```python
from build123d import *

# Parameters (mm, degrees)
CHANFREIN1_SIZE           = 0.5
CHANFREIN2_SIZE           = 1
TROU_TARAUD_M8X1_01_D     = 7
TROU_TARAUD_M8X1_01_DEPTH = 23
TROU_TARAUD_M8X1_01_TIP   = 2.103012167


with BuildPart() as part:
    # Esquisse1 → Révolution1 (revolve)
    with BuildSketch(Plane.XY, mode=Mode.PRIVATE) as r_volution1_sk:
        Polygon((-44, 23), (-13, 23), (-13, 20), (13, 20), (13, 18), (56, 18), (56, 17), (60.5, 17), (60.5, 12.5), (76.5, 12.5), (76.5, 0), (-44, 0), align=None)
    revolve(r_volution1_sk.sketch.rotate(Axis((-47.210983023, 0, 0), (1, 0, 0)), 90), axis=Axis((-47.210983023, 0, 0), (1, 0, 0)))

    # Chanfrein1
    chanfrein1_edges = [part.edges().sort_by_distance(p)[0] for p in [
        (56, 0, -18),
        (13, 0, -20),
        (-13, 0, -23),
    ]]
    chamfer(chanfrein1_edges, length=CHANFREIN1_SIZE)

    # Chanfrein2
    chanfrein2_edges = [part.edges().sort_by_distance(p)[0] for p in [
        (76.5, 0, -12.5),
    ]]
    chamfer(chanfrein2_edges, length=CHANFREIN2_SIZE)

    # Trou taraudé M8x1.01
    with Locations(Plane(origin=(76.5, 0, 0), x_dir=(0, 0, -1), z_dir=(1, 0, 0))):
        with Locations((0, 0)):
            Hole(TROU_TARAUD_M8X1_01_D / 2, depth=TROU_TARAUD_M8X1_01_DEPTH)
            with Locations((0, 0, -(TROU_TARAUD_M8X1_01_DEPTH + TROU_TARAUD_M8X1_01_TIP / 2))):  # 118° drill point
                Cone(0, TROU_TARAUD_M8X1_01_D / 2, TROU_TARAUD_M8X1_01_TIP, mode=Mode.SUBTRACT)


solid = part.part
```
Can you work these out from the model? Positions are in its coordinate system, mm. A direction names the side the tool comes from. Coordinates: 2 decimals unless noted, no trailing zeros. Order: outer loops, then holes, each group sorted by start corner. A loop starts at its lowest first (then second) coordinate and runs counter-clockwise, first axis right, second up. Notation, with made-up numbers: (71.5, 20.5) -> (77.5, 20.5) arc R30 cw to (77.5, 42.5) -> close; hole circle Ø10 at (23, 70.25). An arc over 180 degrees is marked (long way). Write each question's results on one line, items separated by ' | '.
Item 1: Which directions (+Z, -Z, +X, -X, +Y, -Y) give clear straight access to the entire face, cutting with the end or side of a thin tool? Please do faces 4 (the face through (58.282, -16.855, -2.213)), 5 (the face through (76.5, -3, -3)).
Results are:
face 4: +X | face 5: +Z, -Z, +X, +Y, -Y
Item 2: I'm going to push flat-ended pins straight in: pin 1 Ø1 at (x, y) = (-4.5, -2.5) entering from +Z; pin 2 Ø8 at (x, z) = (30, 6) entering from -Y; pin 3 Ø12 at (x, y) = (10.5, 1) entering from +Z. Where does each tip first touch, or does it pass through?
Results are:
pin 1: z = 19.9 | pin 2: y = -17.89 | pin 3: z = 20
Item 3: If I drill on line 1 along Y through (x, z) = (58.25, 0); line 2 along Y through (x, z) = (62, 0); line 3 along X through (y, z) = (-7.5, 20.5), over which ranges is the centre line in solid material (lowest first)?
Results are:
line 1: -17 to -3.5, 3.5 to 17 | line 2: -12.5 to -3.5, 3.5 to 12.5 | line 3: -44 to -13
Item 4: If we mould it in two halves opening along Y, with no side actions, what happens to faces 1 (the face through (64.839, -1.341, 3.233)), 2 (the face through (-28.536, -22.804, -2.994)), 3 (the face through (-13, 1.6, -20.1))? For each: +Y half, -Y half, draft (parallel to the pull), parting line (faces both ways), or undercut.
Results are:
face 1: undercut | face 2: parting line | face 3: draft
Item 5: I want a section at A-A, the plane x = 24. Write out the boundary of the cut face in (y, z).
Results are:
outline: circle Ø36 at (0, 0)
Item 6: I want a section at B-B, the plane x = -18.5. Write out the boundary of the cut face in (y, z), then the cut area to 3 significant figures.
Results are:
outline: circle Ø46 at (0, 0) | area: 1,660 mm²
